from build123d import *

# Parameters (mm, degrees)
SKETCH1_W           = 100
SKETCH1_H           = 120
BOSS_EXTRUDE1_DEPTH = 5
SKETCH2_W           = 100
SKETCH2_H           = 120
SKETCH2_W_2         = 94
SKETCH2_H_2         = 114
BOSS_EXTRUDE2_DEPTH = 40
SKETCH3_W           = 40.8
SKETCH3_H           = 9.2
BOSS_EXTRUDE3_DEPTH = 10
SKETCH4_W           = 114
SKETCH4_H           = 40
BOSS_EXTRUDE4_DEPTH = 15
SKETCH5_R           = 5.3
CUT_EXTRUDE1_DEPTH  = 18
SKETCH8_R           = 1.6
CUT_EXTRUDE2_DEPTH  = 88.749643874
CUT_EXTRUDE3_DEPTH  = 3
SKETCH10_W          = 114
SKETCH10_H          = 37.223183771
BOSS_EXTRUDE6_DEPTH = 3
SKETCH11_R          = 1.4
CUT_EXTRUDE4_DEPTH  = 40
SKETCH14_W          = 12.8
SKETCH14_H          = 15
CUT_EXTRUDE5_DEPTH  = 5
CUT_EXTRUDE6_DEPTH  = 2


with BuildPart() as part:
    # Sketch1 → Boss-Extrude1 (new body)
    with BuildSketch(Plane(origin=(0, 0, 0), x_dir=(1, 0, 0), z_dir=(0, 1, 0))):
        Rectangle(SKETCH1_W, SKETCH1_H)
    extrude(amount=BOSS_EXTRUDE1_DEPTH)

    # Sketch2 → Boss-Extrude2 (add)
    with BuildSketch(Plane(origin=(0, 5, 0), x_dir=(1, 0, 0), z_dir=(0, 1, 0))):
        Rectangle(SKETCH2_W, SKETCH2_H)
        Rectangle(SKETCH2_W_2, SKETCH2_H_2, mode=Mode.SUBTRACT)
    extrude(amount=BOSS_EXTRUDE2_DEPTH)

    # Sketch3 → Boss-Extrude3 (add)
    with BuildSketch(Plane(origin=(0, 5, 0), x_dir=(1, 0, 0), z_dir=(0, 1, 0))):
        with Locations((0, 40)):
            Rectangle(SKETCH3_W, SKETCH3_H)
        Rectangle(SKETCH3_W, SKETCH3_H)
        with Locations((0, -40)):
            Rectangle(SKETCH3_W, SKETCH3_H)
    extrude(amount=BOSS_EXTRUDE3_DEPTH)

    # Sketch4 → Boss-Extrude4 (add)
    with BuildSketch(Plane.ZY.offset(-47)):
        with Locations((0, 25)):
            Rectangle(SKETCH4_W, SKETCH4_H)
    extrude(amount=BOSS_EXTRUDE4_DEPTH)

    # Sketch5 → Cut-Extrude1 (cut)
    with BuildSketch(Plane.ZY.offset(-32)):
        with Locations((-40, 27)):
            Circle(SKETCH5_R)
        with Locations((0, 27)):
            Circle(SKETCH5_R)
        with Locations((40, 27)):
            Circle(SKETCH5_R)
    extrude(amount=-CUT_EXTRUDE1_DEPTH, mode=Mode.SUBTRACT)

    # Sketch8 → Cut-Extrude2 (cut, through all)
    with BuildSketch(Plane(origin=(0, 5, 0), x_dir=(1, 0, 0), z_dir=(0, 1, 0))):
        with Locations(Location((-7.5, -20, 0), (0, 0, 270))):
            Circle(SKETCH8_R)
        with Locations(Location((-7.5, 20, 0), (0, 0, 270))):
            Circle(SKETCH8_R)
    extrude(amount=-CUT_EXTRUDE2_DEPTH, mode=Mode.SUBTRACT)

    # Sketch9 → Cut-Extrude3 (cut)
    with BuildSketch(Plane(origin=(0, 5, 0), x_dir=(1, 0, 0), z_dir=(0, 1, 0))):
        Polygon((-10.271281292, -21.6), (-7.5, -23.2), (-4.728718708, -21.6), (-4.728718708, -18.4), (-7.5, -16.8), (-10.271281292, -18.4), align=None)
        Polygon((-10.271281292, 21.6), (-10.271281292, 18.4), (-7.5, 16.8), (-4.728718708, 18.4), (-4.728718708, 21.6), (-7.5, 23.2), align=None)
    extrude(amount=-CUT_EXTRUDE3_DEPTH, mode=Mode.SUBTRACT)

    # Sketch10 → Boss-Extrude6 (add)
    with BuildSketch(Plane(origin=(-47, 0, 0), x_dir=(0, 0, -1), z_dir=(1, 0, 0))):
        with Locations((0, 26.388408114)):
            Rectangle(SKETCH10_W, SKETCH10_H)
    extrude(amount=BOSS_EXTRUDE6_DEPTH)

    # Sketch11 → Cut-Extrude4 (cut)
    with BuildSketch(Plane(origin=(0, 45, 0), x_dir=(1, 0, 0), z_dir=(0, 1, 0))):
        with Locations(Location((41, -50, 0), (0, 0, 270))):
            Circle(SKETCH11_R)
        with Locations(Location((41, 50, 0), (0, 0, 270))):
            Circle(SKETCH11_R)
        with Locations(Location((-47, 50, 0), (0, 0, 270))):
            Circle(SKETCH11_R)
        with Locations(Location((-47, -50, 0), (0, 0, 270))):
            Circle(SKETCH11_R)
    extrude(amount=-CUT_EXTRUDE4_DEPTH, mode=Mode.SUBTRACT)

    # Sketch14 → Cut-Extrude5 (cut)
    with BuildSketch(Plane.XZ):
        with Locations((24, 20)):
            Rectangle(SKETCH14_W, SKETCH14_H)
    extrude(amount=-CUT_EXTRUDE5_DEPTH, mode=Mode.SUBTRACT)

    # Sketch15 → Cut-Extrude6 (cut)
    with BuildSketch(Plane(origin=(0, 5, 0), x_dir=(1, 0, 0), z_dir=(0, 1, 0))):
        Polygon((30.4, -12.5), (30.4, -8.5), (8.4, -8.5), (8.4, -31.5), (30.4, -31.5), (30.4, -27.5), (17.6, -27.5), (17.6, -12.5), align=None)
    extrude(amount=-CUT_EXTRUDE6_DEPTH, mode=Mode.SUBTRACT)


solid = part.part
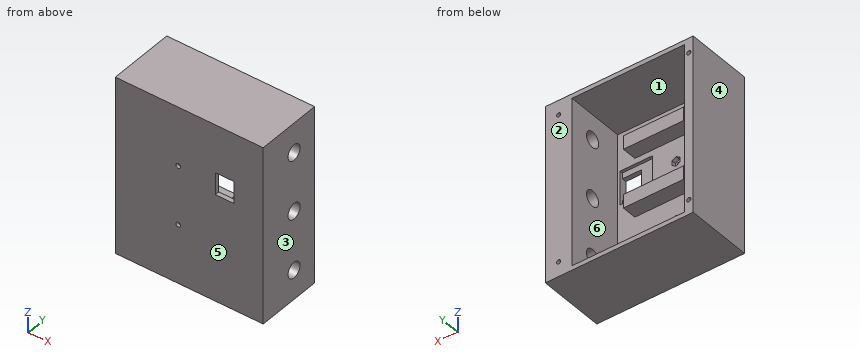
Source: CAD feature listing. Evaluate the final solid. Frame: model axes, mm. Face numbers are marked on the shaded views. A direction names the side the tool comes from. Give positions to 0.01 mm unless a question says otherwise; leave off trailing zeros. Write each loop counter-clockwise with the first axis right and the second up, starting at its lowest first coordinate (ties: lowest second). Pieces come first, ordered by that corner, then holes. Notation, with made-up numbers: (82.5, -8) -> (88.5, -8) arc R10 ccw to (88.5, 4) -> close; hole circle Ø4 at (-36.75, -2.75). An arc over 180 degrees is marked (long way). Return JSON: item names as keys, results as strings. Group by question number.
1. Section C-C, the plane y = 38.5. Output: boundary loops of the cut face in (x, z), then the cut area to 3 significant figures.
2. Material intervals for line 1 (X direction, y = 13.5, z = 0.5); line 2 (Z direction, x = -29, y = 33); line 3 (X direction, y = 18, z = 26.5), sorted ascending. Write a range as from..to.
3. Section D-D, the plane z = 20. Output: boundary loops of the cut face in (x, y).
4. Mould query, pull axis X, two halves, no side actions, for the marked faces 1, 2, 3 and 4. Classes: +X half, -X half, draft (parallel to the pull), parting line (faces both ways), or undercut.
5. Pin query (flat end, axial travel): pin 1 Ø4.5 at (x, z) = (-7.5, 19) entering from +Y; pin 2 Ø3 at (x, z) = (-0.5, -38) entering from +Y; pin 3 Ø4 at (x, z) = (-24.5, 39) entering from -Y. Return the tip coordinate at first contact, or that it passes through.
6. Section A-A, the plane z = 40. Output: boundary loops of the cut face in (x, y).
7. Section B-B, the plane y = 27. Output: boundary loops of the cut face in (x, z).
8. Access query for the marked faces 5 and 6. Directions: +Z, -Z, +X, -X, +Y, -Y. A direction counts if a zero-diameter tool reaches every point of the face in a straight line with its end or side. Return the directions, or none.
Determined:
{
 "1": {"outline": "(-50, -60) -> (50, -60) -> (50, 60) -> (-50, 60) -> close; hole circle Ø2.8 at (-47, -50); hole circle Ø2.8 at (-47, 50); hole (-44, -57) -> (32, -57) -> (32, 57) -> (-44, 57) -> close; hole circle Ø2.8 at (41, -50); hole circle Ø2.8 at (41, 50)", "area": "3,310 mm2"},
 "2": {"line 1": "x = -50..-44, -20.4..20.4, 32..50", "line 2": "z = -60..-57, 57..60", "line 3": "x = -50..-44, 32..50"},
 "3": {"outline": "(-50, 0) -> (-9.1, 0) -> (-9.1, 2) -> (-10.27, 2) -> (-10.27, 5) -> (-47, 5) -> (-47, 7.78) -> (-44, 7.78) -> (-44, 45) -> (-50, 45) -> close; (-5.9, 0) -> (17.6, 0) -> (17.6, 3) -> (8.4, 3) -> (8.4, 5) -> (-4.73, 5) -> (-4.73, 2) -> (-5.9, 2) -> close; (30.4, 0) -> (50, 0) -> (50, 45) -> (32, 45) -> (32, 5) -> (30.4, 5) -> close"},
 "4": {"face 1": "undercut", "face 2": "draft", "face 3": "+X half", "face 4": "-X half"},
 "5": {"pin 1": "stops at y = 5", "pin 2": "stops at y = 15", "pin 3": "stops at y = 0"},
 "6": {"outline": "(-50, 0) -> (50, 0) -> (50, 21.7) -> (32, 21.7) -> (32, 5) -> (20.4, 5) -> (20.4, 15) -> (-20.4, 15) -> (-20.4, 5) -> (-47, 5) -> (-47, 7.78) -> (-44, 7.78) -> (-44, 45) -> (-50, 45) -> close; (32, 32.3) -> (50, 32.3) -> (50, 45) -> (32, 45) -> close"},
 "7": {"outline": "(-50, -60) -> (50, -60) -> (50, -45.3) -> (32, -45.3) -> (32, -57) -> (-44, -57) -> (-44, 57) -> (32, 57) -> (32, 45.3) -> (50, 45.3) -> (50, 60) -> (-50, 60) -> close; (32, -34.7) -> (50, -34.7) -> (50, -5.3) -> (32, -5.3) -> close; (32, 5.3) -> (50, 5.3) -> (50, 34.7) -> (32, 34.7) -> close; hole circle Ø2.8 at (-47, -50); hole circle Ø2.8 at (-47, 50); hole circle Ø2.8 at (41, -50); hole circle Ø2.8 at (41, 50)"},
 "8": {"face 5": "+Z, -Z, +X, -X, -Y", "face 6": "+Y"}
}
